Check sheet for the modelled part. Datum: model origin and axes. Units: mm. Coordinates: 2 decimals unless noted, no trailing zeros. Loops run counter-clockwise (first coordinate to the right, second up) from the corner with the lowest first, then second, coordinate; pieces in that order, holes last. Notation, with made-up numbers: (85.5, 21) - (98.5, 21) arc R12 cw to (98.5, 41) - close; hole circle Ø3 at (65, 34). An arc over 180 degrees is marked (long way). Answer as a JSON object with one key per item and string values. Group by question number.
from build123d import *

# Parameters (mm, degrees)
SKETCH1_W           = 273
SKETCH1_H           = 275
SKETCH1_R           = 75
SKETCH1_W_2         = 223
SKETCH1_H_2         = 47
BOSS_EXTRUDE1_DEPTH = 5
SKETCH2_R           = 5.1
SKETCH2_R_2         = 1.75
SKETCH2_R_3         = 10.5
SKETCH2_R_4         = 2.25
CUT_EXTRUDE1_DEPTH  = 10


with BuildPart() as part:
    # Sketch1 → Boss-Extrude1 (new body)
    with BuildSketch(Plane(origin=(0, 0, 0), x_dir=(1, 0, 0), z_dir=(0, 1, 0))):
        with Locations((136.5, 137.5)):
            Rectangle(SKETCH1_W, SKETCH1_H)
        with Locations((136.5, 137.5)):
            Circle(SKETCH1_R, mode=Mode.SUBTRACT)
        with Locations((136.5, 298.5)):
            Rectangle(SKETCH1_W_2, SKETCH1_H_2)
    extrude(amount=BOSS_EXTRUDE1_DEPTH)

    # Sketch2 → Cut-Extrude1 (cut)
    with BuildSketch(Plane(origin=(0, 5, 0), x_dir=(1, 0, 0), z_dir=(0, 1, 0))):
        with Locations((136.5, 295)):
            Circle(SKETCH2_R)
        with Locations((136.5, 303)):
            Circle(SKETCH2_R_2)
        with Locations((136.5, 287)):
            Circle(SKETCH2_R_2)
        with Locations((128.5, 295)):
            Circle(SKETCH2_R_2)
        with Locations((144.5, 295)):
            Circle(SKETCH2_R_2)
        with Locations((69.38, 303)):
            Circle(SKETCH2_R_3)
        with Locations((80.693708499, 314.313708499)):
            Circle(SKETCH2_R_4)
        with Locations((58.066291501, 314.313708499)):
            Circle(SKETCH2_R_4)
        with Locations((80.693708499, 291.686291501)):
            Circle(SKETCH2_R_4)
        with Locations((58.066291501, 291.686291501)):
            Circle(SKETCH2_R_4)
        with Locations((203.62, 303)):
            Circle(SKETCH2_R_3)
        with Locations((214.933708499, 291.686291501)):
            Circle(SKETCH2_R_4)
        with Locations((192.306291501, 291.686291501)):
            Circle(SKETCH2_R_4)
        with Locations((192.306291501, 314.313708499)):
            Circle(SKETCH2_R_4)
        with Locations((214.933708499, 314.313708499)):
            Circle(SKETCH2_R_4)
    extrude(amount=-CUT_EXTRUDE1_DEPTH, mode=Mode.SUBTRACT)


solid = part.part
1. Material ranges on line 1 (Z direction, x = 136.5, y = 3.45); line 2 (X direction, y = 1.5, z = -303); line 3 (X direction, y = 1.45, z = -136.5), recorded low to high.
2. Release check for a two-part mould opening along X. For faces 1 (the face through (74, 0, -199)), 2 (the face through (67.1, 2.54, -292.75)), 3 (the face through (213.32, 2.54, -298.98)) record: released by +X, released by -X, zero draft, split by the parting line, or undercut.
3. Sectioned sample at A-A on z = -137.5. Record the cut outline in (x, y).
4. Gauge pin test, flat ends, axial feed: pin 1 (3 mm diameter, centred on x = 136.5, z = -287, fed in from +Y); pin 2 (2.5 mm diameter, centred on y = 1.5, z = -294, fed in from +X); pin 3 (2.5 mm diameter, centred on x = 255.5, y = 3, fed in from -Z). Record the tip position at first contact, or that the pin passes through.
5. Sectioned sample at C-C on y = 1.45. State how many separate pieces and enclosed holes the cut face has, plus the area to 3 significant figures.
6. Sectioned sample at B-B on x = 118.5. Record the cut outline in (y, z), plus the area to 3 significant figures.
Answers follow:
{
 "1": {"line 1": "z = -322 to -304.75, -301.25 to -300.1, -289.9 to -288.75, -285.25 to -212.5, -62.5 to 0", "line 2": "x = 25 to 58.88, 79.88 to 134.75, 138.25 to 193.12, 214.12 to 248", "line 3": "x = 0 to 61.51, 211.49 to 273"},
 "2": {"face 1": "zero draft", "face 2": "undercut", "face 3": "undercut"},
 "3": {"outline": "(0, 0) - (61.5, 0) - (61.5, 5) - (0, 5) - close; (211.5, 0) - (273, 0) - (273, 5) - (211.5, 5) - close"},
 "4": {"pin 1": "passes through", "pin 2": "stops at x = 248", "pin 3": "stops at z = -275"},
 "5": {"separate pieces": "1", "enclosed holes": "16", "area": "66,900 mm^2"},
 "6": {"outline": "(0, -322) - (5, -322) - (5, -210.31) - (0, -210.31) - close; (0, -64.69) - (5, -64.69) - (5, 0) - (0, 0) - close", "area": "882 mm^2"}
}
